```python
from build123d import *

# Parameters (mm, degrees)
SCHIZZO1_R                   = 7
ESTRUSIONE_ESTRUSIONE1_DEPTH = 43.6
RIVOLUZIONE1_ANGLE           = 180
RIVOLUZIONE2_ANGLE           = 180


with BuildPart() as part:
    # Schizzo1 → Estrusione-Estrusione1 (new body)
    with BuildSketch(Plane(origin=(0, 0, 0), x_dir=(1, 0, 0), z_dir=(0, 1, 0))):
        with Locations(Location((0, 0, 0), (0, 0, 270))):
            Circle(SCHIZZO1_R)
    extrude(amount=ESTRUSIONE_ESTRUSIONE1_DEPTH)

    # Schizzo2 → Rivoluzione1 (revolve)
    with BuildSketch(Plane(origin=(0, 0, 0), x_dir=(-1, 0, 0), z_dir=(0, -1, 0))):
        with BuildLine():
            Line((-0.415700634, -6.98764574), (0.415700634, 6.98764574))
            ThreePointArc((0.415700634, 6.98764574), (-6.98764574, 0.415700634), (-0.415700634, -6.98764574))
        make_face()
    revolve(axis=Axis((0.415700634, 0, 6.98764574), (-0.05938580489346364, 0, -0.9982351056625666)), revolution_arc=RIVOLUZIONE1_ANGLE)

    # Schizzo3 → Rivoluzione2 (revolve)
    with BuildSketch(Plane(origin=(0, 43.6, 0), x_dir=(1, 0, 0), z_dir=(0, 1, 0))):
        with BuildLine():
            Line((7, 0), (-7, 0))
            ThreePointArc((-7, 0), (0, -7), (7, 0))
        make_face()
    revolve(axis=Axis((7, 43.6, 0), (-1, 0, 0)), revolution_arc=RIVOLUZIONE2_ANGLE)


solid = part.part
```
CAD build for the part. Positions are in the model's coordinates, mm. Round coordinates to 2 decimals unless told otherwise and drop trailing zeros. Write each loop counter-clockwise with the first axis right and the second up, starting at its lowest first coordinate (ties: lowest second). Pieces come first, ordered by that corner, then holes. Notation, with made-up numbers: (44, -8.5) -> (55, -8.5) arc R22 ccw to (55, 8.5) -> close; hole circle Ø2 at (69.25, 39). An arc over 180 degrees is marked (long way). Answer in a Markdown table with one row per item. Add a question column.
Item 1: Saw through at A-A, the plane y = 40.5. Write the cut outline in (x, z).
Item 2: Saw through at B-B, the plane z = 0. Write the cut outline in (x, y), then the cut area to 3 significant figures.
Item 3: Drill centre lines: line 1 (Z direction, x = -6.25, y = 14.5); line 2 (X direction, y = 23, z = 4.75); line 3 (Z direction, x = 2.5, y = -1). Where is each one in solid material? Low to high. Write a range as from..to.
Item 4: Saw through at C-C, the plane x = 5.5. Write the cut outline in (y, z), then the cut area to 3 significant figures.
Item 5: Drop flat-ended pins along their axis: pin 1 Ø1.5 at (x, z) = (-2, 0.5) entering from +Y; pin 2 Ø1.5 at (x, y) = (0.5, 44.5) entering from -Z; pin 3 Ø3 at (x, z) = (2, 3.5) entering from +Y. Give the stop position or say it passes through.
Findings below:
| question | item | result |
|---|---|---|
| 1 | outline | circle Ø14 at (0, 0) |
| 2 | outline | (-7, 0) arc R7 ccw to (7, 0) -> (7, 43.6) arc R7 ccw to (-7, 43.6) -> close |
| 2 | area | 764 mm^2 |
| 3 | line 1 | z = -3.15..3.15 |
| 3 | line 2 | x = -5.14..5.14 |
| 3 | line 3 | z = -6.46..6.46 |
| 4 | outline | (0, -4.33) -> (43.6, -4.33) arc R4.33 ccw to (43.6, 4.33) -> (0, 4.33) arc R4.33 ccw to start |
| 4 | area | 436 mm^2 |
| 5 | pin 1 | stops at y = 50.48 |
| 5 | pin 2 | stops at z = -6.99 |
| 5 | pin 3 | stops at y = 50.13 |
